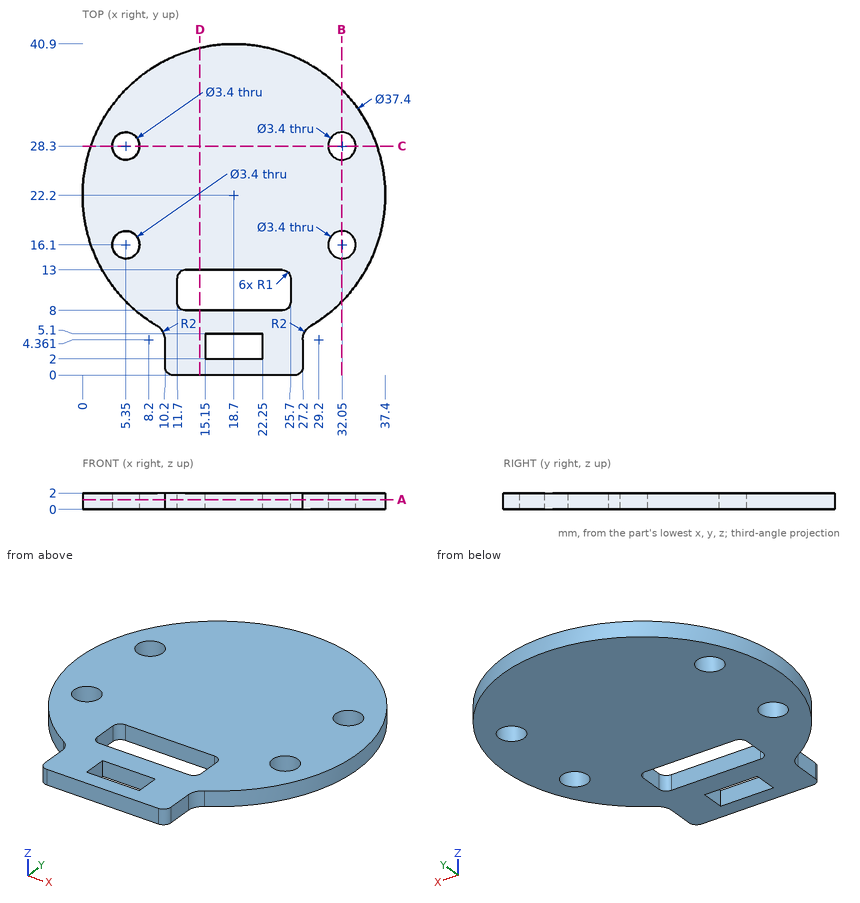
Geometry: see drawing. Coordinates: mm, zero at the bounding-box minimum. Round coordinates to 2 decimals unless told otherwise and drop trailing zeros. Loops run counter-clockwise (first coordinate to the right, second up) from the corner with the lowest first, then second, coordinate; pieces in that order, holes last. Notation, with made-up numbers: (17, 15.25) -> (41, 15.25) arc R21 ccw to (41, 27.25) -> close; hole circle Ø3 at (38, 1). An arc over 180 degrees is marked (long way). Use one line per item in the form item = value. Start each with the question number.
Item 1: Material intervals for L1, parallel to X at y = 4, z = 0.45; L2, parallel to X at y = 17.5, z = 1 (1 decimal); L3, parallel to Y at x = 20, z = 0.9 (1 decimal), sorted ascending. Write a range as from..to.
Item 2: Contact query for flat-ended pins moving along their axis: pin 1 Ø0.6 at (y, z) = (3.5, 0.5) entering from +X; pin 2 Ø2 at (x, y) = (5.35, 16.1) entering from +Z (3 decimals); pin 3 Ø0.6 at (x, z) = (17, 1) entering from +Y; pin 4 Ø1 at (y, z) = (11, 0.5) entering from -X. Output: stop coordinate, or through.
Item 3: Section query B-B on x = 32. Return the cut outline in (y, z) (1 decimal).
Item 4: Section query A-A on z = 1.2. Count the separate pieces of the cut face and the enclosed holes in it, then the cut area to 3 significant figures.
Item 5: Section query D-D on x = 14.5. Return the cut outline in (y, z).
Item 6: Section query C-C on y = 28.3. Return the cut outline in (x, z).
Ans:
q1.L1 = 10.2..15.15, 22.25..27.2
q1.L2 = 0.6..4.4, 6.3..31.1, 33..36.8
q1.L3 = 0..2, 5.1..8, 13..40.9
q2.pin_1 = 27.2
q2.pin_2 = through
q2.pin_3 = 40.85
q2.pin_4 = 3.36
q3.outline = (9.1, 0) -> (14.4, 0) -> (14.4, 2) -> (9.1, 2) -> close; (17.8, 0) -> (26.6, 0) -> (26.6, 2) -> (17.8, 2) -> close; (30, 0) -> (35.3, 0) -> (35.3, 2) -> (30, 2) -> close
q4.separate_pieces = 1
q4.enclosed_holes = 6
q4.area = 1,040 mm^2
q5.outline = (0, 0) -> (8, 0) -> (8, 2) -> (0, 2) -> close; (13, 0) -> (40.42, 0) -> (40.42, 2) -> (13, 2) -> close
q6.outline = (1.02, 0) -> (3.65, 0) -> (3.65, 2) -> (1.02, 2) -> close; (7.05, 0) -> (30.35, 0) -> (30.35, 2) -> (7.05, 2) -> close; (33.75, 0) -> (36.38, 0) -> (36.38, 2) -> (33.75, 2) -> close
